For this review, take the finished solid that the model builds, in its own axes (mm). A direction names the side the tool comes from. Round coordinates to 2 decimals unless told otherwise and drop trailing zeros. Loops run counter-clockwise (first coordinate to the right, second up) from the corner with the lowest first, then second, coordinate; pieces in that order, holes last.
1) Wall thickness on L1, parallel to Y at x = 37.5, z = 27; L2, parallel to Y at x = 13.5, z = 11; L3, parallel to Z at x = 28.5, y = -36: over which ranges is each line inside the solid? List them lowest first.
2) Insertion check: pin 1 (1 mm diameter, centred on y = 37.5, z = 18, fed in from +X); pin 2 (16 mm diameter, centred on x = 17.5, z = 24, fed in from +Y); pin 3 (2 mm diameter, centred on x = 37, z = 35.5, fed in from -Y). Each pin has a flat end and moves straight along its axis. Give the tip position at first contact, or say it passes through.
3) Take a section at B-B (y = 55.5). State the section outline as (x, z) points, then the cut area to 3 significant figures.
4) Take a section at C-C (x = 5.5). State the section outline as (y, z) points, then the cut area to 3 significant figures.
5) Tool access review of faces 1 (the cylindrical face through (44.145, 57.402, 10.829)), 2 (the cylindrical face through (44.14, 38.4, 19.01)), 3 (the flat face through (22, -45.5, 27)): name each direction out of +Z, -Z, +X, -X, +Y, -Y from which nothing blocks a thin tool from reaching the whole face with its end or side.
6) Mouldability with a two-part tool opening along Y and no side actions: class faces 4 (the cylindrical face through (44.14, -44.6, 26.59)), 5 (the flat face through (22, 58.5, 8)), 6 (the cylindrical face through (0.9, 66.64, 6.27)) as pulls with the +Y half, pulls with the -Y half, needs draft (parallel to the pull), parting line crosses it, or undercut.
7) Take a section at D-D (x = 27). State the section outline as (y, z) points.
8) Take a section at A-A (z = 29). State the section outline as (x, y) points, then the cut area to 3 significant figures.
Autodesk Inventor part; units mm, degrees
ref_plane "YZ Plane" through (0, 0, 0) normal (1, 0, 0) x (0, 1, 0)
ref_plane "XZ Plane" through (0, 0, 0) normal (0, 1, 0) x (-1, 0, 0)
ref_plane "XY Plane" through (0, 0, 0) normal (0, 0, 1) x (1, 0, 0)
sketch "Sketch1" plane through (0, 0, 0) normal (1, 0, 0) x (0, 1, 0)
  line L0 (-67.5, 3.7308) -> (-37.5, 3.7308)
  line L1 (-37.5, 3.7308) -> (-37.5, 31.7308)
  line L2 (-37.5, 31.7308) -> (37.5, 31.7308)
  line L3 (37.5, 31.7308) -> (37.5, 3.7308)
  line L4 (37.5, 3.7308) -> (67.5, 3.7308)
  line L5 (67.5, 3.7308) -> (67.5, 11.7308)
  line L6 (67.5, 11.7308) -> (45.5, 11.7308)
  line L7 (45.5, 11.7308) -> (45.5, 39.7308)
  line L8 (45.5, 39.7308) -> (-45.5, 39.7308)
  line L9 (-45.5, 39.7308) -> (-45.5, 11.7308)
  line L10 (-45.5, 11.7308) -> (-67.5, 11.7308)
  line L11 (-67.5, 11.7308) -> (-67.5, 3.7308)
  line L12 (0, 0) -> (0, 98)
  dimension "d0" = 75
  dimension "d1" = 30
  dimension "d2" = 8
  dimension "d3" = 8
  dimension "d4" = 8
  dimension "d5" = 8
  dimension "d6" = 28
extrude "Extrusion1" add sketch "Sketch1" along normal blind 45
sketch "Sketch2" plane through (0, 45.5, 11.7308) normal (0, 0, 1) x (1, 0, 0)
  line L0 (0, -45.5) -> (80, -45.5)
  line L1 (0, 22) -> (0, 0)
  line L2 (0, 0) -> (45, 0)
  line L3 (45, 22) -> (45, 0)
  line L4 (0, 22) -> (45, 22)
  line L5 (32, 10) -> (13, 10) construction
  line L6 (32, 7) -> (13, 7)
  line L7 (13, 13) -> (32, 13)
  arc A0 (32, 7) -> (32, 13) centre (32, 10) ccw
  arc A1 (13, 13) -> (13, 7) centre (13, 10) ccw
  line L8 (32, -98) -> (13, -98)
  line L9 (13, -104) -> (32, -104)
  arc A2 (32, -104) -> (32, -98) centre (32, -101) ccw
  arc A3 (13, -98) -> (13, -104) centre (13, -101) ccw
  point P0 (22.5, 10)
extrude "Extrusion2" cut sketch "Sketch2" against normal through all contours L6 A1 L7 A0 | A2 L9 A3 L8
fillet "Fillet1" radius 5 2 edges at (22.5, 45.5, 11.7308) (22.5, -45.5, 11.7308)
fillet "Fillet2" radius 3 24 edges at (22.5, 45.5, 39.7308) (0, 0, 39.7308) (0, 37.5, 17.7308) (0, 0, 31.7308) (0, -37.5, 17.7308) (0, -59, 11.7308) (0, -45.5, 28.2308) (45, 0, 39.7308) (45, 59, 11.7308) (45, 45.5, 28.2308) (0, 59, 11.7308) (0, 45.5, 28.2308) (22.5, 67.5, 11.7308) (45, 67.5, 7.7308) (0, 67.5, 7.7308) (22.5, -45.5, 39.7308) (22.5, -67.5, 11.7308) (0, -67.5, 7.7308) (45, -67.5, 7.7308) (45, -59, 11.7308) (45, -45.5, 28.2308) (45, -37.5, 17.7308) (45, 0, 31.7308) (45, 37.5, 17.7308)
properties part number "sujeta-taladro-0,1"
Response:
1. L1: y = -45.5 to -37.5, 37.5 to 45.5
1. L2: y = -66.46 to -58.5, -52.5 to -37.5, 37.5 to 52.5, 58.5 to 66.46
1. L3: z = 31.73 to 39.73
2. pin 1: stops at x = 43.66
2. pin 2: stops at y = 45.55
2. pin 3: stops at y = -45.5
3. outline: (0, 3.73) - (10, 3.73) - (10, 11.73) - (3, 11.73) arc R3 ccw to (0, 8.73) - close; (35, 3.73) - (45, 3.73) - (45, 8.73) arc R3 ccw to (42, 11.73) - (35, 11.73) - close
3. area: 156 mm2
4. outline: (-67.5, 3.73) - (-37.5, 3.73) - (-37.5, 31.73) - (37.5, 31.73) - (37.5, 3.73) - (67.5, 3.73) - (67.5, 8.73) arc R3 ccw to (64.5, 11.73) - (50.5, 11.73) arc R5 cw to (45.5, 16.73) - (45.5, 36.73) arc R3 ccw to (42.5, 39.73) - (-42.5, 39.73) arc R3 ccw to (-45.5, 36.73) - (-45.5, 16.73) arc R5 cw to (-50.5, 11.73) - (-64.5, 11.73) arc R3 ccw to (-67.5, 8.73) - close
4. area: 1,530 mm2
5. face 1: +Z, +X, +Y
5. face 2: -Z, +X
5. face 3: +Z, +X, -X, -Y
6. face 4: pulls with the -Y half
6. face 5: undercut
6. face 6: pulls with the +Y half
7. outline: (-67.5, 3.73) - (-58.5, 3.73) - (-58.5, 11.73) - (-64.5, 11.73) arc R3 ccw to (-67.5, 8.73) - close; (-52.5, 3.73) - (-37.5, 3.73) - (-37.5, 31.73) - (37.5, 31.73) - (37.5, 3.73) - (52.5, 3.73) - (52.5, 11.73) - (50.5, 11.73) arc R5 cw to (45.5, 16.73) - (45.5, 36.73) arc R3 ccw to (42.5, 39.73) - (-42.5, 39.73) arc R3 ccw to (-45.5, 36.73) - (-45.5, 16.73) arc R5 cw to (-50.5, 11.73) - (-52.5, 11.73) - close; (58.5, 3.73) - (67.5, 3.73) - (67.5, 8.73) arc R3 ccw to (64.5, 11.73) - (58.5, 11.73) - close
8. outline: (0, -42.5) arc R3 ccw to (3, -45.5) - (42, -45.5) arc R3 ccw to (45, -42.5) - (45, -40.5) arc R3 ccw to (42, -37.5) - (3, -37.5) arc R3 ccw to (0, -40.5) - close; (0, 40.5) arc R3 ccw to (3, 37.5) - (42, 37.5) arc R3 ccw to (45, 40.5) - (45, 42.5) arc R3 ccw to (42, 45.5) - (3, 45.5) arc R3 ccw to (0, 42.5) - close
8. area: 705 mm2
